```python
from build123d import *

# Parameters (mm, degrees)
SKETCH1_R           = 6
SKETCH1_R_2         = 3
BOSS_EXTRUDE1_DEPTH = 11
SKETCH2_R           = 1.5
CUT_EXTRUDE1_DEPTH  = 14.892443989
SKETCH3_R           = 6
BOSS_EXTRUDE2_DEPTH = 4
BOSS_EXTRUDE3_DEPTH = 7
SKETCH5_R           = 3
BOSS_EXTRUDE6_DEPTH = 14
SKETCH7_R           = 2.5
BOSS_EXTRUDE7_DEPTH = 5
FILLET1_R           = 0.5
ECHELLE1_SCALE      = 2
ECHELLE2_SCALE      = 0.25


with BuildPart() as part:
    # Sketch1 → Boss-Extrude1 (new body)
    with BuildSketch(Plane.XY):
        Circle(SKETCH1_R)
        Circle(SKETCH1_R_2, mode=Mode.SUBTRACT)
    extrude(amount=BOSS_EXTRUDE1_DEPTH)

    # Sketch2 → Cut-Extrude1 (cut, through all)
    with BuildSketch(Plane(origin=(0, 0, 0), x_dir=(1, 0, 0), z_dir=(0, 1, 0))):
        with Locations(Location((0, -6, 0), (0, 0, 90))):
            Circle(SKETCH2_R)
    extrude(amount=CUT_EXTRUDE1_DEPTH, mode=Mode.SUBTRACT)

    # Sketch3 → Boss-Extrude2 (add)
    with BuildSketch(Plane.XY.offset(11)):
        Circle(SKETCH3_R)
    extrude(amount=BOSS_EXTRUDE2_DEPTH)

    # Sketch4 → Boss-Extrude3 (add)
    with BuildSketch(Plane.XY.offset(15)):
        with BuildLine():
            Line((-1.658312395, 2.5), (1.658312395, 2.5))
            ThreePointArc((1.658312395, 2.5), (0, -3), (-1.658312395, 2.5))
        make_face()
    extrude(amount=BOSS_EXTRUDE3_DEPTH)

    # Sketch5 → Boss-Extrude6 (add)
    with BuildSketch(Plane.XY.offset(22)):
        Circle(SKETCH5_R)
    extrude(amount=BOSS_EXTRUDE6_DEPTH)

    # Sketch7 → Boss-Extrude7 (add)
    with BuildSketch(Plane.XY.offset(36)):
        Circle(SKETCH7_R)
    extrude(amount=BOSS_EXTRUDE7_DEPTH)

    # Fillet1
    fillet1_edges = [part.edges().sort_by_distance(p)[0] for p in [
        (0, -3, 15),
    ]]
    fillet(fillet1_edges, radius=FILLET1_R)


with BuildPart() as part_1:
    # Echelle1: scaled about (-5.064e-06, -0.057271287, 14.482309023)
    add(part.part.scale(ECHELLE1_SCALE).moved(Location((5.064e-06, 0.057271287, -14.482309023))))


with BuildPart() as part_2:
    # Echelle2: scaled about (-5.063e-06, -0.057271287, 14.482309023)
    add(part_1.part.scale(ECHELLE2_SCALE).moved(Location((-3.797e-06, -0.042953465, 10.861731767))))


solid = part_2.part
```
Design review of the part built by this model. Coordinates are the model's own, in mm. A direction names the side the tool comes from. Coordinates: 2 decimals unless noted, no trailing zeros. Write each loop counter-clockwise with the first axis right and the second up, starting at its lowest first coordinate (ties: lowest second). Pieces come first, ordered by that corner, then holes.
1) To check wall thickness, follow L1, parallel to X at y = 0, z = 11; L2, parallel to Z at x = -0.5, y = 0; L3, parallel to Z at x = 0.5, y = 2.5. State the ranges of each line that lie inside material, in increasing order.
2) Mouldability with a two-part tool opening along X and no side actions: class faces 1 (the cylindrical face through (-0.225, 2.11, 9.526)), 2 (the cylindrical face through (-0.3, -1.5, 10)), 3 (the flat face through (0, 1.221, 16)), 4 (the cylindrical face through (-1.25, 0.03, 26.47)) as +X half, -X half, draft (parallel to the pull), parting line (faces both ways), or undercut.
3) Insertion check: pin 1 (0.9 mm diameter, centred on x = 0, z = 10.24, fed in from +Y); pin 2 (2 mm diameter, centred on x = -0.5, z = 16.5, fed in from +Y); pin 3 (1.5 mm diameter, centred on x = 1.5, z = 20.5, fed in from -Y). Each pin has a flat end and moves straight along its axis. Give the tip position at first contact, or say it passes through.
4) Machinability: for faces 5 (the flat face through (0, 0, 12.741)), 6 (the flat face through (0, 0, 27.741)), which of the approach directions +Z, -Z, +X, -X, +Y, -Y give a long, thin tool a straight path to every point of the face, cutting with its end or side? Answer none if there is none.
5) Add section B-B (y = 2). Write out the cut boundary in (x, z).
6) Add section C-C (z = 12). Write out the cut boundary in (x, y).
7) Add section A-A (z = 17.25). Write out the cut boundary in (x, y).
8) Add section D-D (x = 2.5). Write out the cut boundary in (y, z), plus the area to 3 significant figures.
Check result:
1. L1: x = -3 to -1.5, 1.5 to 3
1. L2: z = 12.74 to 27.74
1. L3: z = 7.24 to 9.68, 10.8 to 14.74
2. face 1: undercut
2. face 2: undercut
2. face 3: draft
2. face 4: parting line
3. pin 1: stops at y = -1.46
3. pin 2: stops at y = 1.22
3. pin 3: stops at y = -1.33
4. face 5: -Z
4. face 6: +Z, +X, -X, +Y, -Y
5. outline: (-2.21, 7.24) - (2.21, 7.24) - (2.21, 14.74) - (-2.21, 14.74) - close; hole circle Ø1.5 at (0, 10.24)
6. outline: circle Ø6 at (0, -0.03); hole circle Ø3 at (0, -0.03)
7. outline: (-0.83, 1.22) arc R1.5 ccw (long way) to (0.83, 1.22) - close
8. outline: (-1.69, 7.24) - (1.63, 7.24) - (1.63, 14.74) - (-1.69, 14.74) - close
8. area: 24.9 mm2
